from build123d import *

# Parameters (mm, degrees)
M3_TAPPED_HOLE1_D = 2.5
CIRPATTERN1_COUNT = 4


with BuildPart() as part:
    # Sketch1 → Revolve1 (revolve)
    with BuildSketch(Plane(origin=(0, 0, 0), x_dir=(0, 0, -1), z_dir=(1, 0, 0))):
        Polygon((1.6, 0), (1.6, 1), (2.93, 1), (2.93, 4.5), (4.5, 4.5), (4.5, 2.5), (10, 2.5), (10, 0), align=None)
    revolve(axis=Axis((0, 0, 0), (0, 1, 0)))

    # M3 Tapped Hole1 (through all)
    with Locations(Plane(origin=(0, 0, 0), x_dir=(-1, 0, 0), z_dir=(0, -1, 0))):
        with Locations((0, -7)):
            m3_tapped_hole1 = Hole(M3_TAPPED_HOLE1_D / 2)

    # CirPattern1: M3 Tapped Hole1 ×4 about axis
    cirpattern1_axis = Axis((0, 0, 0), (0, 1, 0))
    for i in range(1, CIRPATTERN1_COUNT):
        add(m3_tapped_hole1.rotate(cirpattern1_axis, i * 360 / CIRPATTERN1_COUNT), mode=Mode.SUBTRACT)


solid = part.part
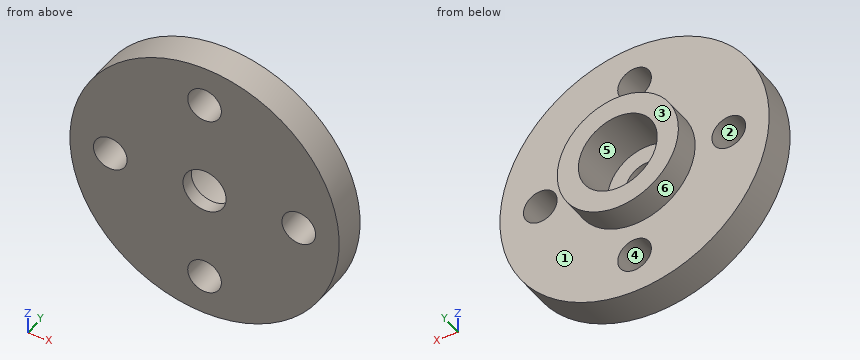
The listing builds one solid part. Answer for the finished solid, in the listing's coordinates (mm). Face numbers are marked on the shaded views. A direction names the side the tool comes from. Round coordinates to 2 decimals unless told otherwise and drop trailing zeros. Order: outer loops, then holes, each group sorted by start corner. A loop starts at its lowest first (then second) coordinate and runs counter-clockwise, first axis right, second up. Notation, with made-up numbers: (72, 17.25) -> (88, 17.25) arc R23 cw to (88, 46.25) -> close; hole circle Ø3 at (28.25, 30). An arc over 180 degrees is marked (long way). Write each question's results on one line, items separated by ' | '. Start each with the question number.
Q1. Find section B-B (x = 0). Determine the outline of the cut face in (y, z), then the cut area to 3 significant figures.
Q2. Find section A-A (x = 6). Determine the outline of the cut face in (y, z), then the cut area to 4 significant figures.
Q3. Which of the six approach directions +Z, -Z, +X, -X, +Y, -Y give full straight-line access (tool end or side, diameter ignored) to the marked faces 1 and 2?
Q4. Each of these flat-tipped pins is pushed along its axis until it touches: pin 1 (3 mm diameter, centred on x = 0, z = 7, fed in from +Y); pin 2 (1 mm diameter, centred on x = -3.5, y = 2.5, fed in from +Z); pin 3 (4 mm diameter, centred on x = 0, z = 0, fed in from +Y). Where does it stop, or does it pass through?
Q5. Find section C-C (z = -1). Determine the outline of the cut face in (x, y), then the cut area to 3 significant figures.
Q6. Straight lines are drawn through the part: probe 1 along X at (y, z) = (0.75, 0); probe 2 along X at (y, z) = (1.85, 0). For each, find the intervals that lie inside material, in ascending order. Write a range as from..to.
Q7. The mould has two halves that part along X. Classify the marked faces 3, 4, 5 and 6: pulls with the +X half, pulls with the -X half, needs draft (parallel to the pull), parting line crosses it, or undercut.
Q8. Find section D-D (z = 6.5). Determine the outline of the cut face in (x, y).
Worked answers:
1) outline: (0, -10) -> (2.5, -10) -> (2.5, -8.25) -> (0, -8.25) -> close; (0, -5.75) -> (2.5, -5.75) -> (2.5, -4.5) -> (4.5, -4.5) -> (4.5, -2.93) -> (1, -2.93) -> (1, -1.6) -> (0, -1.6) -> close; (0, 1.6) -> (1, 1.6) -> (1, 2.93) -> (4.5, 2.93) -> (4.5, 4.5) -> (2.5, 4.5) -> (2.5, 5.75) -> (0, 5.75) -> close; (0, 8.25) -> (2.5, 8.25) -> (2.5, 10) -> (0, 10) -> close | area: 31.8 mm2
2) outline: (0, -8) -> (2.5, -8) -> (2.5, -0.75) -> (0, -0.75) -> close; (0, 0.75) -> (2.5, 0.75) -> (2.5, 8) -> (0, 8) -> close | area: 36.25 mm2
3) face 1: +Y | face 2: +Y, -Y
4) pin 1: stops at y = 2.5 | pin 2: stops at z = 9.54 | pin 3: stops at y = 1
5) outline: (-9.95, 0) -> (-7.75, 0) -> (-7.75, 2.5) -> (-9.95, 2.5) -> close; (-6.25, 0) -> (-1.25, 0) -> (-1.25, 1) -> (-2.75, 1) -> (-2.75, 4.5) -> (-4.39, 4.5) -> (-4.39, 2.5) -> (-6.25, 2.5) -> close; (1.25, 0) -> (6.25, 0) -> (6.25, 2.5) -> (4.39, 2.5) -> (4.39, 4.5) -> (2.75, 4.5) -> (2.75, 1) -> (1.25, 1) -> close; (7.75, 0) -> (9.95, 0) -> (9.95, 2.5) -> (7.75, 2.5) -> close | area: 38.0 mm2
6) probe 1: x = -10..-8.25, -5.75..-1.6, 1.6..5.75, 8.25..10 | probe 2: x = -10..-8.25, -5.75..-2.93, 2.93..5.75, 8.25..10
7) face 3: needs draft | face 4: undercut | face 5: undercut | face 6: parting line crosses it
8) outline: (-7.6, 0) -> (-1.15, 0) -> (-1.15, 2.5) -> (-7.6, 2.5) -> close; (1.15, 0) -> (7.6, 0) -> (7.6, 2.5) -> (1.15, 2.5) -> close
